The listing builds one solid part. Answer for the finished solid, in the listing's coordinates (mm). A direction names the side the tool comes from. Give positions to 0.01 mm unless a question says otherwise; leave off trailing zeros. Loops run counter-clockwise (first coordinate to the right, second up) from the corner with the lowest first, then second, coordinate; pieces in that order, holes last. Notation, with made-up numbers: M 38.25,89 L 55.25,89 A21 ccw 55.25,98 Z; hole C -2,-18 d11. An arc over 180 degrees is marked long. Use one line per item in the form item = value. Start each with the question number.
1. The part is cut by section C-C (y = -9.5). Write down the section's boundary in (x, z), and give its area (3 significant figures).
2. The part is cut by section B-B (z = 1.1). Write down the section's boundary in (x, y), and give its area (3 significant figures).
3. For faces 1 (the face through (27.149, -15, 1)), 2 (the face through (29, 4.068, 1)), 3 (the face through (-17.851, -18, 1)), 4 (the face through (-34, -5.932, 1)), determine the directions among +Z, -Z, +X, -X, +Y, -Y from which every point of the face is accessible in a straight line to the end or side of a thin tool.
4. The part is cut by section A-A (x = 1). Write down the section's boundary in (y, z).
5. Each of these flat-tipped pins is pushed along its axis until it touches: pin 1 Ø6 at (x, y) = (-23.5, -0.5) entering from -Z; pin 2 Ø1.5 at (y, z) = (-18.5, 1.5) entering from -X; pin 3 Ø1.5 at (x, z) = (-34.5, 1) entering from +Y; pin 4 Ø0.9 at (y, z) = (-18, 2) entering from +X. Where does it stop, or does it pass through?
6. Straight lines are drawn through the part: line 1 (X direction, y = -18, z = 1.35); line 2 (Y direction, x = -7, z = 2.45); line 3 (X direction, y = 11.5, z = 2.05). For each, find the intervals that lie inside material, in ascending order. Write a range as from..to.
7. The mould has two halves that part along X. Classify faces 5 (the face through (-3, -4, 0)), 6 (the face through (17, -19.932, 1)), 7 (the face through (-32.851, -14, 1)), 8 (the face through (-3, -19.932, 1)): released by +X, released by -X, zero draft, split by the parting line, or undercut.
from build123d import *

# Parameters (mm, degrees)
SKETCH1_W           = 10
SKETCH1_H           = 3
SKETCH1_W_2         = 3
SKETCH1_H_2         = 10
BOSS_EXTRUDE1_DEPTH = 3


with BuildPart() as part:
    # Sketch1 → Boss-Extrude1 (new body)
    # profile 1 of 4: a face of its own
    with BuildSketch(Plane.XY):
        Polygon((-2.850678733, -16.932126697), (-2.850678733, 15.067873303), (-32.850678733, 15.067873303), (-32.850678733, 4.067873303), (-32.850678733, -5.932126697), (-32.850678733, -22.932126697), (-2.850678733, -22.932126697), (-2.850678733, -19.932126697), (-7.850678733, -19.932126697), (-7.850678733, -16.932126697), align=None)
        with Locations((-22.850678733, -18.432126697)):
            Rectangle(SKETCH1_W, SKETCH1_H, mode=Mode.SUBTRACT)
    # profile 2 of 4: a face of its own
    with BuildSketch(Plane.XY):
        Polygon((27.149321267, 15.067873303), (-2.850678733, 15.067873303), (-2.850678733, -16.932126697), (2.149321267, -16.932126697), (2.149321267, -19.932126697), (-2.850678733, -19.932126697), (-2.850678733, -22.932126697), (27.149321267, -22.932126697), (27.149321267, -5.932126697), (27.149321267, 4.067873303), align=None)
        with Locations((17.149321267, -18.432126697)):
            Rectangle(SKETCH1_W, SKETCH1_H, mode=Mode.SUBTRACT)
    # profile 3 of 4: a face of its own
    with BuildSketch(Plane.XY):
        with Locations((-34.350678733, -0.932126697)):
            Rectangle(SKETCH1_W_2, SKETCH1_H_2)
    # profile 4 of 4: a face of its own
    with BuildSketch(Plane.XY):
        with Locations((28.649321267, -0.932126697)):
            Rectangle(SKETCH1_W_2, SKETCH1_H_2)
    extrude(amount=BOSS_EXTRUDE1_DEPTH)


solid = part.part
Derived:
q1.outline = M -32.85,0 L 27.15,0 L 27.15,3 L -32.85,3 Z
q1.area = 180 mm2
q2.outline = M -35.85,-5.93 L -32.85,-5.93 L -32.85,-22.93 L 27.15,-22.93 L 27.15,-5.93 L 30.15,-5.93 L 30.15,4.07 L 27.15,4.07 L 27.15,15.07 L -32.85,15.07 L -32.85,4.07 L -35.85,4.07 Z; hole M -27.85,-19.93 L -17.85,-19.93 L -17.85,-16.93 L -27.85,-16.93 Z; hole M -7.85,-19.93 L 2.15,-19.93 L 2.15,-16.93 L -7.85,-16.93 Z; hole M 12.15,-19.93 L 22.15,-19.93 L 22.15,-16.93 L 12.15,-16.93 Z
q2.area = 2,250 mm2
q3.face_1 = +Z, -Z, +X, -Y
q3.face_2 = +Z, -Z, +X, +Y
q3.face_3 = +Z, -Z
q3.face_4 = +Z, -Z, -X, -Y
q4.outline = M -22.93,0 L -19.93,0 L -19.93,3 L -22.93,3 Z; M -16.93,0 L 15.07,0 L 15.07,3 L -16.93,3 Z
q5.pin_1 = 0
q5.pin_2 = -32.85
q5.pin_3 = 4.07
q5.pin_4 = 27.15
q6.line_1 = -32.85..-27.85, -17.85..-7.85, 2.15..12.15, 22.15..27.15
q6.line_2 = -22.93..-19.93, -16.93..15.07
q6.line_3 = -32.85..27.15
q7.face_5 = zero draft
q7.face_6 = undercut
q7.face_7 = released by -X
q7.face_8 = undercut
